Verification items for the finished model (mm, model axes). Face numbers are marked on the shaded views. A direction names the side the tool comes from. Give positions to 0.01 mm unless a question says otherwise; leave off trailing zeros. Order: outer loops, then holes, each group sorted by start corner. A loop starts at its lowest first (then second) coordinate and runs counter-clockwise, first axis right, second up.
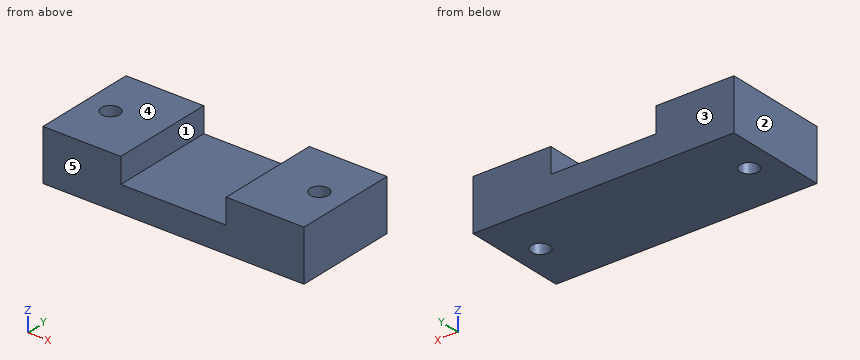
from build123d import *

# Parameters (mm, degrees)
SKETCH2_W           = 50
SKETCH2_H           = 20
SKETCH2_R           = 1.75
BOSS_EXTRUDE1_DEPTH = 5
BOSS_EXTRUDE2_DEPTH = 20
SKETCH6_R           = 1.75
CUT_EXTRUDE1_DEPTH  = 10.8


with BuildPart() as part:
    # Sketch2 → Boss-Extrude1 (new body)
    with BuildSketch(Plane.XY):
        Rectangle(SKETCH2_W, SKETCH2_H)
        with Locations((-20, 0)):
            Circle(SKETCH2_R, mode=Mode.SUBTRACT)
        with Locations((20, 0)):
            Circle(SKETCH2_R, mode=Mode.SUBTRACT)
    extrude(amount=BOSS_EXTRUDE1_DEPTH)

    # Sketch5 → Boss-Extrude2 (add)
    with BuildSketch(Plane.XZ.offset(10)):
        with BuildLine():
            Line((-25, 5), (-25, 9.8))
            Line((-25, 9.8), (-10.1, 9.8))
            Line((-10.1, 9.8), (-10.1, 5))
            Line((-10.1, 5), (10.1, 5))
            Line((10.1, 5), (10.1, 9.8))
            Line((10.1, 9.8), (25, 9.8))
            Line((25, 9.8), (25, 5))
            ThreePointArc((25, 5), (0, 0), (-25, 5))
        make_face()
    extrude(amount=-BOSS_EXTRUDE2_DEPTH)

    # Sketch6 → Cut-Extrude1 (cut, through all)
    with BuildSketch(Plane(origin=(0, 0, 0), x_dir=(-1, 0, 0), z_dir=(0, 0, -1))):
        with Locations((20, 0)):
            Circle(SKETCH6_R)
        with Locations((-20, 0)):
            Circle(SKETCH6_R)
    extrude(amount=-CUT_EXTRUDE1_DEPTH, mode=Mode.SUBTRACT)


solid = part.part
(1) Scan lines: line 1 (Y direction, x = 20, z = 2.6); line 2 (X direction, y = 4.5, z = 7.5); line 3 (Z direction, x = 4, y = -2). Record each from-to range of solid material in increasing order.
Solved:
line 1: y = -10 to -1.75, 1.75 to 10
line 2: x = -25 to -10.1, 10.1 to 25
line 3: z = 0 to 5
(2) Section check D-D, the plane y = -2.5. Enter the section's corners in (x, z).
Solved:
outline: (-25, 0) - (25, 0) - (25, 9.8) - (10.1, 9.8) - (10.1, 5) - (-10.1, 5) - (-10.1, 9.8) - (-25, 9.8) - close
(3) Go/stop test with a flat-tipped pin: pin 1 (6 mm diameter, centred on x = 3.5, y = -4, fed in from +Z). Record where the tip stops, or that it passes through.
Solved:
pin 1: stops at z = 5
(4) Section check A-A, the plane z = 7.25. Enter the section's corners in (x, y).
Solved:
outline: (-25, -10) - (-10.1, -10) - (-10.1, 10) - (-25, 10) - close; (10.1, -10) - (25, -10) - (25, 10) - (10.1, 10) - close; hole circle Ø3.5 at (-20, 0); hole circle Ø3.5 at (20, 0)
(5) Set-up check for the marked faces 1 and 2: record each of +Z, -Z, +X, -X, +Y, -Y from which the full face is reachable in a straight line by a thin tool's end or side.
Solved:
face 1: +Z, +Y, -Y
face 2: +Z, -Z, -X, +Y, -Y
(6) Release check for a two-part mould opening along Y. For the marked faces 3, 4 and 5 record: pulls with the +Y half, pulls with the -Y half, needs draft (parallel to the pull), parting line crosses it, or undercut.
Solved:
face 3: pulls with the +Y half
face 4: needs draft
face 5: pulls with the -Y half
(7) Section check B-B, the plane x = 20. Enter the section's corners in (y, z).
Solved:
outline: (-10, 0) - (-1.75, 0) - (-1.75, 9.8) - (-10, 9.8) - close; (1.75, 0) - (10, 0) - (10, 9.8) - (1.75, 9.8) - close
(8) Section check C-C, the plane y = 0. Enter the section's corners in (x, z).
Solved:
outline: (-25, 0) - (-21.75, 0) - (-21.75, 9.8) - (-25, 9.8) - close; (-18.25, 0) - (18.25, 0) - (18.25, 9.8) - (10.1, 9.8) - (10.1, 5) - (-10.1, 5) - (-10.1, 9.8) - (-18.25, 9.8) - close; (21.75, 0) - (25, 0) - (25, 9.8) - (21.75, 9.8) - close
